```python
from build123d import *

# Parameters (mm, degrees)
F2_W     = 2.55
F2_H     = 14.264992
F3_DEPTH = 6.5
F4_SIZE  = 1


with BuildPart() as f1:
    # F0 (on Front) → F1 (revolve)
    with BuildSketch(Plane.XZ):
        Polygon((0, 11.25), (0, 0), (39, 0), (39, 4.975), (21.5, 4.975), (21.5, 4.995), (6.5, 4.995), (6.5, 11.25), align=None)
    revolve(axis=Axis((19.5, 0, 0), (1, 0, 0)))

    # F2 (on face) → F3 (cut, through all)
    with BuildSketch(Plane(origin=(0, 0, 0), x_dir=(0, -1, 0), z_dir=(-1, 0, 0))):
        with Locations((-9.975, 0)):
            Rectangle(F2_W, F2_H)
        with Locations((9.975, 0)):
            Rectangle(F2_W, F2_H)
    extrude(amount=-F3_DEPTH, mode=Mode.SUBTRACT)

    # F4
    f4_edges = [f1.edges().sort_by_distance(p)[0] for p in [
        (39, 0, -4.975),
    ]]
    chamfer(f4_edges, length=F4_SIZE)


solid = f1.part
```
Check sheet for the modelled part. Datum: model origin and axes. Units: mm. A direction names the side the tool comes from. Round coordinates to 2 decimals unless told otherwise and drop trailing zeros. Loops run counter-clockwise (first coordinate to the right, second up) from the corner with the lowest first, then second, coordinate; pieces in that order, holes last. Notation, with made-up numbers: (72, -11) - (102, -11) arc R23 ccw to (102, 4) - close; hole circle Ø10 at (-28, -20). An arc over 180 degrees is marked (long way). Answer as a JSON object with one key per item and string values. Group by question number.
Q1. Sectioned sample at A-A, the plane z = 0. Enter the section's corners in (x, y) (3 decimals).
Q2. Sectioned sample at C-C, the plane x = 20. Enter the section's corners in (y, z) (3 decimals), plus the area to 3 significant figures.
Q3. Gauge pin test, flat ends, axial feed: P1, Ø1, axis at y = -0.5, z = 9, coming from the +X side; P2, Ø6, axis at x = 16, y = -3, coming from the -Z side (3 decimals); P3, Ø5, axis at x = 31.5, z = -0.5, coming from the -Y side (3 decimals). Record the tip position at first contact, or that the pin passes through.
Q4. Sectioned sample at D-D, the plane x = 28.5. Enter the section's corners in (y, z) (3 decimals).
Q5. Set-up check for faces 1 (the face through (3, 8.7, 0)), 2 (the face through (29.634, 3.027, -3.948)): record each of +Z, -Z, +X, -X, +Y, -Y from which the full face is reachable in a straight line by a thin tool's end or side.
Q6. Sectioned sample at B-B, the plane y = 0. Enter the section's corners in (x, z) (3 decimals).
Q7. Scan lines: line 1 along X through (y, z) = (5.75, -8.25); line 2 along Z through (x, y) = (18.5, -0.5); line 3 along Y through (x, z) = (34.5, -3). Record each from-to range of solid material in increasing order. Write a range as [from, to].
Solution:
{
 "1": {"outline": "(0, -8.7) - (6.5, -8.7) - (6.5, -4.995) - (21.5, -4.995) - (21.5, -4.975) - (38, -4.975) - (39, -3.975) - (39, 3.975) - (38, 4.975) - (21.5, 4.975) - (21.5, 4.995) - (6.5, 4.995) - (6.5, 8.7) - (0, 8.7) - close"},
 "2": {"outline": "circle Ø9.99 at (0, 0)", "area": "78.4 mm²"},
 "3": {"P1": "stops at x = 6.5", "P2": "stops at z = -4.995", "P3": "stops at y = -4.975"},
 "4": {"outline": "circle Ø9.95 at (0, 0)"},
 "5": {"face 1": "+Z, -Z, +X, -X, +Y", "face 2": "+X"},
 "6": {"outline": "(0, -11.25) - (6.5, -11.25) - (6.5, -4.995) - (21.5, -4.995) - (21.5, -4.975) - (38, -4.975) - (39, -3.975) - (39, 3.975) - (38, 4.975) - (21.5, 4.975) - (21.5, 4.995) - (6.5, 4.995) - (6.5, 11.25) - (0, 11.25) - close"},
 "7": {"line 1": "x = [0, 6.5]", "line 2": "z = [-4.97, 4.97]", "line 3": "y = [-3.97, 3.97]"}
}
